```python
from build123d import *

# Parameters (mm, degrees)
CROQUIS1_R                                           = 40
SALIENTE_EXTRUIR2_DEPTH                              = 50
SALIENTE_EXTRUIR3_DEPTH                              = 80
SALIENTE_EXTRUIR4_DEPTH                              = 20
REFRENTADO_PARA_TORNILLO_CON_CABEZA_TRON_D           = 16
REFRENTADO_PARA_TORNILLO_CON_CABEZA_TRON_CBORE_D     = 28
REFRENTADO_PARA_TORNILLO_CON_CABEZA_TRON_CBORE_DEPTH = 20


with BuildPart() as part:
    # Croquis1 → Saliente-Extruir2 (new body)
    with BuildSketch(Plane.XY):
        with BuildLine():
            ThreePointArc((-187.0195, 177.123901659), (-252.9805, 177.123901659), (-285.961, 120))
            ThreePointArc((-285.961, 120), (-269.616671449, 76.536918708), (-228.683534972, 54.613076679))
            ThreePointArc((-228.683534972, 54.613076679), (-222.477877617, 51.289318393), (-220, 44.700109422))
            Line((-220, 44.700109422), (-220, 30))
            ThreePointArc((-220, 30), (-217.071067812, 22.928932188), (-210, 20))
            Line((-210, 20), (-154.641016151, 20))
            Line((-154.641016151, 20), (-30, -51.961524227))
            ThreePointArc((-30, -51.961524227), (-52.868956993, 28.370290561), (26.713161338, 53.725292101))
            Line((26.713161338, 53.725292101), (-187.0195, 177.123901659))
        make_face()
        with BuildLine():
            ThreePointArc((-72.471012114, 12.973644893), (-69.725821585, 2.728454364), (-79.971012114, -0.016736164))
            Line((-79.971012114, -0.016736164), (-166.573552492, 49.983263836))
            ThreePointArc((-166.573552492, 49.983263836), (-169.31874302, 60.228454364), (-159.073552492, 62.973644893))
            Line((-159.073552492, 62.973644893), (-72.471012114, 12.973644893))
        make_face(mode=Mode.SUBTRACT)
        with BuildLine():
            ThreePointArc((-56.25, 41.069262024), (-53.504809472, 30.824071495), (-63.75, 28.078880967))
            Line((-63.75, 28.078880967), (-150.352540378, 78.078880967))
            ThreePointArc((-150.352540378, 78.078880967), (-153.097730907, 88.324071495), (-142.852540378, 91.069262024))
            Line((-142.852540378, 91.069262024), (-56.25, 41.069262024))
        make_face(mode=Mode.SUBTRACT)
        with Locations((-220, 120)):
            Circle(CROQUIS1_R, mode=Mode.SUBTRACT)
        with BuildLine():
            ThreePointArc((-40.028987886, 69.164879154), (-37.283797358, 58.919688626), (-47.528987886, 56.174498098))
            Line((-47.528987886, 56.174498098), (-134.131528265, 106.174498098))
            ThreePointArc((-134.131528265, 106.174498098), (-136.876718793, 116.419688626), (-126.631528265, 119.164879154))
            Line((-126.631528265, 119.164879154), (-40.028987886, 69.164879154))
        make_face(mode=Mode.SUBTRACT)
    extrude(amount=SALIENTE_EXTRUIR2_DEPTH)

    # Croquis1_4 → Saliente-Extruir3 (add)
    with BuildSketch(Plane.XY):
        with BuildLine():
            Line((33.166247904, 50), (80, 50))
            Line((80, 50), (80, 4))
            Line((80, 4), (39.799497484, 4))
            ThreePointArc((39.799497484, 4), (-40, 0), (39.799497484, -4))
            Line((39.799497484, -4), (80, -4))
            Line((80, -4), (80, -50))
            Line((80, -50), (33.166247904, -50))
            ThreePointArc((33.166247904, -50), (-60, 0), (33.166247904, 50))
        make_face()
    extrude(amount=SALIENTE_EXTRUIR3_DEPTH)

    # Croquis1_5 → Saliente-Extruir4 (add)
    with BuildSketch(Plane.XY):
        with BuildLine():
            ThreePointArc((-228.683534972, 54.613076679), (-269.616671449, 76.536918708), (-285.961, 120))
            Line((-285.961, 120), (-285.961, 40))
            ThreePointArc((-285.961, 40), (-280.103135624, 25.857864376), (-265.961, 20))
            Line((-265.961, 20), (-210, 20))
            ThreePointArc((-210, 20), (-217.071067812, 22.928932188), (-220, 30))
            Line((-220, 30), (-220, 44.700109422))
            ThreePointArc((-220, 44.700109422), (-222.477877617, 51.289318393), (-228.683534972, 54.613076679))
        make_face()
    extrude(amount=SALIENTE_EXTRUIR4_DEPTH)

    # Refrentado para tornillo con cabeza tron (through all)
    with Locations(Plane(origin=(56.583, 50, 60), x_dir=(0, 0, 1), z_dir=(0, 1, 0))):
        with Locations((0, 0), (-40, 0.726384558)):
            CounterBoreHole(REFRENTADO_PARA_TORNILLO_CON_CABEZA_TRON_D / 2, REFRENTADO_PARA_TORNILLO_CON_CABEZA_TRON_CBORE_D / 2, REFRENTADO_PARA_TORNILLO_CON_CABEZA_TRON_CBORE_DEPTH)


solid = part.part
```
Part model, mm, in its own coordinate system. A direction names the side the tool comes from. Coordinates: 2 decimals unless noted, no trailing zeros. Loops run counter-clockwise (first coordinate to the right, second up) from the corner with the lowest first, then second, coordinate; pieces in that order, holes last. Notation, with made-up numbers: (64, 20.25) - (105, 20.25) arc R15 ccw to (105, 40.25) - close; hole circle Ø5 at (-34.5, -35.5). An arc over 180 degrees is marked (long way). Write item = value, one per line. Start each with the question number.
Item 1: Flat gauge pins, fed straight in: pin 1 Ø6 at (x, z) = (-28, 48) entering from +Y; pin 2 Ø2 at (y, z) = (-29, 14) entering from -X; pin 3 Ø6 at (x, z) = (-197.5, 24.5) entering from +Y. Where does each tip first touch, or does it go through?
Item 2: Wall check: L1, parallel to X at y = -33, z = 25; L2, parallel to Y at x = 0, z = 44; L3, parallel to X at y = 74.5, z = 21. Give the ranges that are in metal, low to high. Write a range as from..to.
Item 3: Cut at B-B, the plane z = 58. Give the cut face in (x, y), and give its area (3 significant figures).
Item 4: Cut at C-C, the plane x = -105. Give the cut face in (y, z), and give its area (3 significant figures).
Item 5: 3-axis set-ups, long thin cutter, end or side, ignore diameter. For faces 1 (the cylindrical face through (61.515, 40.14, 33.354)), 2 (the flat face through (-116.379, 38.324, 24.65)), 3 (the flat face through (60, 4, 39)): which of +Z, -Z, +X, -X, +Y, -Y reach the whole face in a straight line?
Item 6: Cut at D-D, the plane x = -205. Give the cut face in (y, z), and give its area (3 significant figures).
Item 7: Cut at A-A, the plane x = -5. Give the cut face in (y, z), and give its area (3 significant figures).
Item 8: Mould opens along Y. For faces 4 (the flat face through (-122.666, 24.633, 24.65)), 5 (the cylindrical face through (-32.99, -50.116, 57.218)), 6 (the flat face through (51, 30, 26)), 7 (the cylindrical face through (-153.18, 88.18, 24.65)) say: released by +Y, released by -Y, zero draft, split by the parting line, or undercut.
The answers:
q1.pin_1 = 87.05
q1.pin_2 = -71.5
q1.pin_3 = 183.01
q2.L1 = -62.84..-22.61, 22.61..51.06, 63.55..80
q2.L2 = -60..-40, 40..69.15
q2.L3 = -267.76..-144.15, -114.15..-79.27, -49.27..-9.27
q3.outline = (33.17, -50) - (48.84, -50) - (48.84, -4) - (39.8, -4) arc R40 cw (long way) to (39.8, 4) - (48.84, 4) - (48.84, 30) - (42.73, 30) - (42.73, 50) - (33.17, 50) arc R60 ccw (long way) to start; (64.33, -50) - (80, -50) - (80, -4) - (64.33, -4) - close; (64.33, 4) - (80, 4) - (80, 50) - (70.44, 50) - (70.44, 30) - (64.33, 30) - close
q3.area = 7,090 mm2
q4.outline = (-8.66, 0) - (14.43, 0) - (14.43, 50) - (-8.66, 50) - close; (31.75, 0) - (51.89, 0) - (51.89, 50) - (31.75, 50) - close; (69.22, 0) - (89.36, 0) - (89.36, 50) - (69.22, 50) - close; (106.68, 0) - (129.77, 0) - (129.77, 50) - (106.68, 50) - close
q4.area = 4,320 mm2
q5.face_1 = +Y
q5.face_2 = +Z, -Z
q5.face_3 = +Z, -Z, +X
q6.outline = (20, 0) - (82.92, 0) - (82.92, 50) - (20, 50) - close; (157.08, 0) - (184.23, 0) - (184.23, 50) - (157.08, 50) - close
q6.area = 4,500 mm2
q7.outline = (-59.79, 0) - (-39.69, 0) - (-39.69, 80) - (-59.79, 80) - close; (39.69, 0) - (72.03, 0) - (72.03, 50) - (59.79, 50) - (59.79, 80) - (39.69, 80) - close
q7.area = 3,830 mm2
q8.face_4 = undercut
q8.face_5 = split by the parting line
q8.face_6 = released by +Y
q8.face_7 = undercut
